from build123d import *

# Parameters (mm, degrees)
BOSS_EXTRUDE1_DEPTH    = 1.5
SKETCH2_W              = 41
SKETCH2_H              = 40
BOSS_EXTRUDE2_DEPTH    = 1.5
CONVERT_SOLID1_START   = -20
CONVERT_SOLID1_DEPTH   = 40
CONVERT_SOLID1_2_DEPTH = 40
M3_CLEARANCE_HOLE1_D   = 3.2
CIRPATTERN1_COUNT      = 6
CUT_EXTRUDE1_DEPTH     = 54.525694764
M3_CLEARANCE_HOLE2_D   = 3.4
LPATTERN1_COUNT        = 2
LPATTERN1_PITCH        = 24
LPATTERN1_COPY_1_D     = 3.4
FILLET1_R              = 3


# Read off the part's stored shape, not the designer's step: Convert-Solid1
with BuildPart() as part:
    # Sketch1 → Boss-Extrude1 (new body)
    with BuildSketch(Plane(origin=(0, 0, 0), x_dir=(0, 0, -1), z_dir=(1, 0, 0))):
        with BuildLine():
            Line((-20, 0), (-20, -28))
            Line((-20, -28), (20, -28))
            Line((20, -28), (20, 0))
            ThreePointArc((20, 0), (0, 20), (-20, 0))
        make_face()
    extrude(amount=BOSS_EXTRUDE1_DEPTH)

    # Sketch2 → Boss-Extrude2 (add)
    with BuildSketch(Plane.XZ.offset(28)):
        with Locations((20.5, 0)):
            Rectangle(SKETCH2_W, SKETCH2_H)
    extrude(amount=-BOSS_EXTRUDE2_DEPTH)

    # Convert-Solid1 outline → Convert-Solid1 (cut)
    with BuildSketch(Plane.XY.offset(CONVERT_SOLID1_START)):
        with BuildLine():
            Line((0, -28), (2.262, -28))
            ThreePointArc((2.262, -28), (0.662524461, -27.337475539), (0, -25.738))
            Line((0, -25.738), (0, -28))
        make_face()
    extrude(amount=CONVERT_SOLID1_DEPTH, mode=Mode.SUBTRACT)

    # Convert-Solid1 2 outline → Convert-Solid1 2 (add)
    with BuildSketch(Plane.XY.offset(CONVERT_SOLID1_START)):
        with BuildLine():
            Line((1.5, -26.5), (2.262, -26.5))
            ThreePointArc((2.262, -26.5), (1.723184633, -26.276815367), (1.5, -25.738))
            Line((1.5, -25.738), (1.5, -26.5))
        make_face()
    extrude(amount=CONVERT_SOLID1_2_DEPTH)

    # M3 Clearance Hole1 (through all)
    with Locations(Plane.ZY):
        with Locations((-15.5, 0)):
            m3_clearance_hole1 = Hole(M3_CLEARANCE_HOLE1_D / 2)

    # CirPattern1: M3 Clearance Hole1 ×6 about axis
    cirpattern1_axis = Axis((0, 0, 0), (1, 0, 0))
    for i in range(1, CIRPATTERN1_COUNT):
        add(m3_clearance_hole1.rotate(cirpattern1_axis, i * 360 / CIRPATTERN1_COUNT), mode=Mode.SUBTRACT)

    # Sketch9 → Cut-Extrude1 (cut, through all)
    with BuildSketch(Plane.ZY):
        with BuildLine():
            Line((6.5, 7), (6.5, -7))
            ThreePointArc((6.5, -7), (0, -13.5), (-6.5, -7))
            Line((-6.5, -7), (-6.5, 7))
            ThreePointArc((-6.5, 7), (0, 13.5), (6.5, 7))
        make_face()
    extrude(amount=-CUT_EXTRUDE1_DEPTH, mode=Mode.SUBTRACT)

    # M3 Clearance Hole2 (through all)
    with Locations(Plane(origin=(0, -26.5, 0), x_dir=(1, 0, 0), z_dir=(0, 1, 0))):
        with Locations((33, 15)):
            m3_clearance_hole2 = Hole(M3_CLEARANCE_HOLE2_D / 2)

    # Mirror1: M3 Clearance Hole2 across plane
    add(m3_clearance_hole2.mirror(Plane.XY), mode=Mode.SUBTRACT)

    # LPattern1: M3 Clearance Hole2 ×2
    with Locations(*[(-i * LPATTERN1_PITCH, 0, 0) for i in range(1, LPATTERN1_COUNT)]):
        add(m3_clearance_hole2, mode=Mode.SUBTRACT)

    # LPattern1 copy 1 (through all)
    with Locations(Plane(origin=(-24, -26.5, 0), x_dir=(1, 0, 0), z_dir=(0, 1, 0))):
        with Locations((33, -15)):
            Hole(LPATTERN1_COPY_1_D / 2)

    # Fillet1
    fillet1_edges = [part.edges().sort_by_distance(p)[0] for p in [
        (41, -27.25, 20),
        (41, -27.25, -20),
    ]]
    fillet(fillet1_edges, radius=FILLET1_R)


solid = part.part
For this review, take the finished solid that the model builds, in its own axes (mm). A direction names the side the tool comes from. Give positions to 0.01 mm unless a question says otherwise; leave off trailing zeros. Order: outer loops, then holes, each group sorted by start corner. A loop starts at its lowest first (then second) coordinate and runs counter-clockwise, first axis right, second up. Notation, with made-up numbers: (83.25, 36) -> (131.25, 36) arc R17 ccw to (131.25, 45) -> close; hole circle Ø3 at (67, 63.5). An arc over 180 degrees is marked (long way). Write item = value, one per line.
1) We need section A-A, the plane x = 33. Give the boundary of the cut face in (y, z), and give its area (3 significant figures).
Findings:
outline = (-28, -20) -> (-26.5, -20) -> (-26.5, -16.7) -> (-28, -16.7) -> close; (-28, -13.3) -> (-26.5, -13.3) -> (-26.5, 13.3) -> (-28, 13.3) -> close; (-28, 16.7) -> (-26.5, 16.7) -> (-26.5, 20) -> (-28, 20) -> close
area = 49.8 mm^2
2) Insertion check: pin 1 (1.9 mm diameter, centred on y = 0, z = -15.5, fed in from +X); pin 2 (1.2 mm diameter, centred on x = 0.5, y = 2, fed in from -Z); pin 3 (2 mm diameter, centred on y = 13, z = -10.5, fed in from +X); pin 4 (5.5 mm diameter, centred on x = 9, z = 15, fed in from +Y). Each pin has a flat end and moves straight along its axis. Give the tip position at first contact, or say it passes through.
Findings:
pin_1 = through
pin_2 = -19.95
pin_3 = 1.5
pin_4 = -26.5
3) We need section C-C, the plane y = 3. Give the boundary of the cut face in (x, z), and give its area (3 significant figures).
Findings:
outline = (0, -19.77) -> (1.5, -19.77) -> (1.5, -6.5) -> (0, -6.5) -> close; (0, 6.5) -> (1.5, 6.5) -> (1.5, 19.77) -> (0, 19.77) -> close
area = 39.8 mm^2
4) Draft analysis for pull direction Z (two halves, no side actions). For faces 1 (the face through (40.1, -27.24, -19.14)), 2 (the face through (0.76, -11.861, -8.097)), 3 (the face through (1, 20, 0)), 4 (the face through (0, -13, -4)), state which applies: pulls with the +Z half, pulls with the -Z half, needs draft (parallel to the pull), parting line crosses it, or undercut.
Findings:
face_1 = pulls with the -Z half
face_2 = undercut
face_3 = parting line crosses it
face_4 = needs draft
5) We need section B-B, the plane z = 5. Give the boundary of the cut face in (x, y), and give its area (3 significant figures).
Findings:
outline = (0, -25.74) arc R2.26 ccw to (2.26, -28) -> (41, -28) -> (41, -26.5) -> (2.26, -26.5) arc R0.76 cw to (1.5, -25.74) -> (1.5, -11.15) -> (0, -11.15) -> close; (0, 11.15) -> (1.5, 11.15) -> (1.5, 19.36) -> (0, 19.36) -> close
area = 95.9 mm^2
6) For faces 5 (the face through (9.37, -27.26, -13.34)), 6 (the face through (0.7, 13.5, -0.1)), 7 (the face through (21, -26.5, 0)), list the 3-axis set-ups (+Z, -Z, +X, -X, +Y, -Y) from which the entire face can be reached by the end or side of a thin tool; tool diameter is ignored.
Findings:
face_5 = +Y, -Y
face_6 = +X, -X
face_7 = +Z, -Z, +X, +Y
7) To check wall thickness, follow L1, parallel to Y at x = 0.6, z = 7.75; L2, parallel to X at y = -9.5, z = 9; L3, parallel to Y at x = 1, z = 7.75. State the ranges of each line that lie inside material, in increasing order. Write a range as from..to.
Findings:
L1 = -27.27..-15.02, -11.82..11.82, 15.02..18.44
L2 = 0..1.5
L3 = -27.62..-15.02, -11.82..11.82, 15.02..18.44
8) We need section D-D, the plane z = 15. Give the boundary of the cut face in (x, y), and give its area (3 significant figures).
Findings:
outline = (0, -25.74) arc R2.26 ccw to (2.26, -28) -> (7.3, -28) -> (7.3, -26.5) -> (2.26, -26.5) arc R0.76 cw to (1.5, -25.74) -> (1.5, -1.52) -> (0, -1.52) -> close; (0, 1.52) -> (1.5, 1.52) -> (1.5, 13.23) -> (0, 13.23) -> close; (10.7, -28) -> (31.3, -28) -> (31.3, -26.5) -> (10.7, -26.5) -> close; (34.7, -28) -> (41, -28) -> (41, -26.5) -> (34.7, -26.5) -> close
area = 105 mm^2
